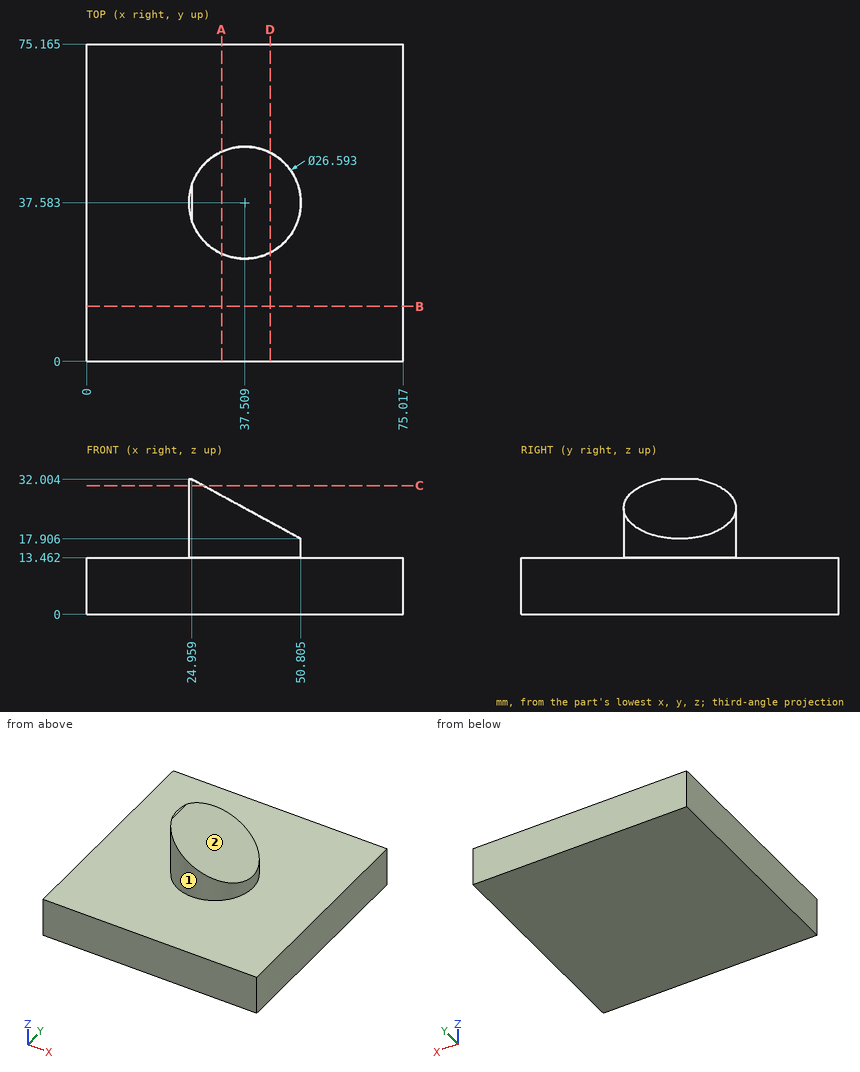
Verification items for this drawing (mm, ordinates from the low corner). A direction names the side the tool comes from. Coordinates: 2 decimals unless noted, no trailing zeros. Order: outer loops, then holes, each group sorted by start corner. A loop starts at its lowest first (then second) coordinate and runs counter-clockwise, first axis right, second up.
Q1. Sectioned sample at D-D on x = 43.5. Record the cut outline in (y, z) (1 decimal).
Reply:
outline: (0, 0) - (75.2, 0) - (75.2, 13.5) - (49.5, 13.5) - (49.5, 21.9) - (25.7, 21.9) - (25.7, 13.5) - (0, 13.5) - close
Q2. Sectioned sample at B-B on y = 13. Record the cut outline in (x, z).
Reply:
outline: (0, 0) - (75.02, 0) - (75.02, 13.46) - (0, 13.46) - close
Q3. Tool access check on the marked faces 1 and 2. Record the directions out of +Z, -Z, +X, -X, +Y, -Y that give a thin tool (end or side, any length) a straight path to the whole face; none if there is none.
Reply:
face 1: +Z
face 2: +Z, +X, +Y, -Y
Q4. Sectioned sample at C-C on z = 30.5. Record the cut outline in (x, y) (1 decimal).
Reply:
outline: (27.7, 28.6) - (27.7, 46.6) arc R13.3 ccw to start
Q5. Depth check by flat-ended pin: pin 1 Ø4 at (x, y) = (67, 16) entering from -Z; pin 2 Ø10 at (x, y) = (53.5, 41.5) entering from +Z; pin 3 Ø4 at (x, z) = (45.5, 22.5) entering from +Y; pin 4 Ø8 at (y, z) = (38.5, 27.5) entering from -X. Enter the tip coordinate at first touch or a pass-through.
Reply:
pin 1: stops at z = 0
pin 2: stops at z = 19.16
pin 3: stops at y = 49.39
pin 4: stops at x = 24.21
Q6. Sectioned sample at A-A on x = 32. Record the cut outline in (y, z) (1 decimal), and give its area (3 significant figures).
Reply:
outline: (0, 0) - (75.2, 0) - (75.2, 13.5) - (49.7, 13.5) - (49.7, 28.2) - (25.5, 28.2) - (25.5, 13.5) - (0, 13.5) - close
area: 1,370 mm2
Q7. Thickness scan on probe 1 along Z at (x, y) = (64, 71); probe 2 along Y at (x, z) = (42, 19.5); probe 3 along X at (y, z) = (28.5, 19) (1 decimal). Record the ranges inside material, lowest first.
Reply:
probe 1: z = 0 to 13.46
probe 2: y = 25.07 to 50.1
probe 3: x = 27.8 to 47.2
